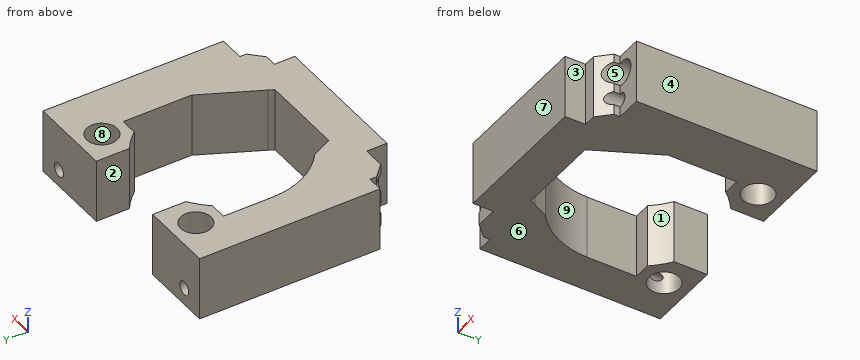
Autodesk Inventor part; units mm, degrees
ref_plane "YZ Plane" through (0, 0, 0) normal (1, 0, 0) x (0, 1, 0)
ref_plane "XZ Plane" through (0, 0, 0) normal (0, 1, 0) x (-1, 0, 0)
ref_plane "XY Plane" through (0, 0, 0) normal (0, 0, 1) x (1, 0, 0)
sketch "Sketch1" plane through (0, 0, 0) normal (0, 0, 1) x (1, 0, 0)
  line L0 (0, 0) -> (50, 0)
  line L1 (50, 0) -> (50, 36.921)
  line L2 (50, 36.921) -> (0, 36.921)
  line L3 (0, 36.921) -> (0, 0)
  dimension "d0" = 36.921
  dimension "d1" = 50
extrude "Extrusion1" add sketch "Sketch1" along normal blind 13
sketch "Sketch4" plane through (0, 0, 0) normal (0, 0, -1) x (-1, 0, 0)
  line L0 (-10, -8) -> (-40, -8)
  line L1 (-45.066, 0) -> (-2.934, 0)
  line L2 (-10.3, -8) -> (-10.3, -3.845)
  line L3 (-10.3, -3.845) -> (-5.7813, -3.845)
  line L4 (-5.7813, -3.845) -> (-3.234, -1.2977)
  line L5 (-3.234, -1.2977) -> (-3.234, 0)
  line L6 (-44.766, 0) -> (-44.766, -1.2977)
  line L7 (-44.766, -1.2977) -> (-42.2187, -3.845)
  line L8 (-42.2187, -3.845) -> (-39.7, -3.845)
  line L9 (-39.7, -3.845) -> (-39.7, -8)
  line L10 (0, 0) -> (-2.934, 0)
  line L11 (0, 0) -> (-50, 0)
  point P0 (-45.066, -1.422)
  dimension "d27" = 2.934
extrude "Extrusion4" add sketch "Sketch4" against normal blind 13
sketch "Sketch2" plane through (0, 0, 0) normal (0, -1, 0) x (1, 0, 0)
  circle A0 centre (44.9, 3.5) radius 1.4
  circle A1 centre (4.9, 3.5) radius 1.4
  line L0 (50, 0) -> (50, 13)
  circle A2 centre (45.7, 9) radius 2.5
  circle A3 centre (4.1, 9) radius 2.5
  line L1 (0, 0) -> (0, 13)
  line L2 (0, 13) -> (50, 13)
  dimension "d4" = 2.8
  dimension "d5" = 2.8
  dimension "d7" = 40
  dimension "d8" = 5
  dimension "d9" = 5
  dimension "d10" = 5.5
  dimension "d13" = 4.1
  dimension "d14" = 5.5
  dimension "d15" = 4
  dimension "d16" = 4.9
  dimension "d17" = 41.6
  dimension "d20" = 4
extrude "Extrusion2" cut sketch "Sketch2" along normal blind 10 and the other way blind 5
sketch "Sketch7" plane through (0, 0, 0) normal (0, 0, -1) x (-1, 0, 0)
  arc A0 (17, 30.1329) -> (13.5279, 26.921) centre (26, 16.921) ccw
  line L0 (10, 26.921) -> (13.5279, 26.921)
  line L1 (10, 12.8998) -> (10, 26.921)
  line L2 (15.8642, 1.1093) -> (10, 12.8998)
  line L3 (16.416, 0) -> (33.6258, 0)
  line L4 (16.416, 0) -> (15.8642, 1.1093)
  line L5 (34.1776, 1.1093) -> (33.6258, 0)
  line L6 (35.7354, 4.2414) -> (34.1776, 1.1093)
  arc A1 (35.7354, 4.2414) -> (41.9856, 16.8076) centre (26, 16.921) ccw
  line L7 (42, 26.921) -> (42, 16.8366)
  line L8 (38.4721, 26.921) -> (42, 26.921)
  arc A2 (38.4721, 26.921) -> (35, 30.1328) centre (26, 16.921) ccw
  line L9 (35, 36.921) -> (35, 30.1328)
  line L10 (17, 30.1329) -> (17, 36.921)
  circle A3 centre (11, 31.921) radius 3.1
  circle A4 centre (41, 31.921) radius 3.1
  line L11 (42, 16.8366) -> (41.9856, 16.8076)
  line L12 (17, 36.921) -> (35, 36.921)
  line L13 (17, 35.9386) -> (35, 35.9386)
  line L14 (35, 35.9386) -> (35, 37.4386)
  line L15 (35, 37.4386) -> (17, 37.4386)
  line L16 (17, 37.4386) -> (17, 35.9386)
  line L17 (0, 36.921) -> (0, 0)
  line L18 (0, 36.921) -> (-15, 36.921)
  line L19 (0, 36.921) -> (15, 36.921) construction
  line L20 (-33, 35.9386) -> (-15, 35.9386)
  line L21 (-33, 36.921) -> (-15, 36.921)
  line L22 (-15, 37.4386) -> (-33, 37.4386)
  line L23 (-33, 37.4386) -> (-33, 35.9386)
  line L24 (-33, 30.1329) -> (-33, 36.921)
  arc A5 (-33, 30.1329) -> (-36.4721, 26.921) centre (-24, 16.921) ccw
  circle A6 centre (-39, 31.921) radius 3.1
  line L25 (-40, 26.921) -> (-36.4721, 26.921)
  line L26 (-40, 12.8998) -> (-40, 26.921)
  line L27 (-34.1358, 1.1093) -> (-40, 12.8998)
  line L28 (-33.584, 0) -> (-16.3742, 0)
  line L29 (-33.584, 0) -> (-34.1358, 1.1093)
  line L30 (-8, 16.8366) -> (-8.0144, 16.8076)
  arc A7 (-14.2646, 4.2414) -> (-8.0144, 16.8076) centre (-24, 16.921) ccw
  line L31 (-14.2646, 4.2414) -> (-15.8224, 1.1093)
  line L32 (-15.8224, 1.1093) -> (-16.3742, 0)
  line L33 (-8, 26.921) -> (-8, 16.8366)
  line L34 (-15, 35.9386) -> (-15, 37.4386)
  arc A8 (-11.5279, 26.921) -> (-15, 30.1328) centre (-24, 16.921) ccw
  line L35 (-11.5279, 26.921) -> (-8, 26.921)
  circle A9 centre (-9, 31.921) radius 3.1
  line L36 (-15, 36.921) -> (-15, 30.1328)
  point P0 (-35, 36.921)
  dimension "d33" = 1.5
  dimension "d34" = 15
  dimension "d35" = 180
  dimension "d39" = 1.5
extrude "Extrusion7" cut sketch "Sketch7" against normal blind 13 contours L23 L21 L34 L20 | L20 L36 A8 L35 L33 L30 A7 L31 L32 L28 L29 L27 L26 L25 A5 L24 | L23 L22 L34 L21 | A6 | A9
sketch "Sketch8" plane through (0, 36.921, 13) normal (0, 1, 0) x (1, 0, 0)
  circle A0 centre (4.9, 9.5) radius 1.4
  circle A1 centre (44.9, 9.5) radius 1.4
  point P0 (0, 13)
extrude "Extrusion8" cut sketch "Sketch8" against normal blind 10
properties part number "30_CUBE_openSIM_Rodholder"
Design review of the part built by this model. Coordinates are the model's own, in mm. Face numbers are marked on the shaded views. A direction names the side the tool comes from. Coordinates: 2 decimals unless noted, no trailing zeros. Write each loop counter-clockwise with the first axis right and the second up, starting at its lowest first coordinate (ties: lowest second). Pieces come first, ordered by that corner, then holes. Notation, with made-up numbers: (-9, -35) - (19, -35) arc R32 cw to (19, -8) - close; hole circle Ø10 at (81, 0.5). An arc over 180 degrees is marked (long way). One line per item, written item: value.
1) Add section B-B (x = 13.5). State the section outline as (y, z) points, plus the area to 3 significant figures.
Answer sheet:
outline: (-8, 0) - (4.87, 0) - (4.87, 13) - (-8, 13) - close; (28.98, 0) - (36.92, 0) - (36.92, 13) - (28.98, 13) - close
area: 271 mm2
2) Add section C-C (x = 45.7). State the section outline as (y, z) points.
Answer sheet:
outline: (0, 0) - (36.92, 0) - (36.92, 2.35) - (26.92, 2.35) - (26.92, 4.65) - (36.92, 4.65) - (36.92, 13) - (0, 13) - (0, 11.5) - (5, 11.5) - (5, 6.5) - (0, 6.5) - (0, 4.65) - (5, 4.65) - (5, 2.35) - (0, 2.35) - close
3) To check wall thickness, follow probe 1 along X at (y, z) = (17.5, 8.75); probe 2 along Y at (x, z) = (11, 7); probe 3 along Y at (x, z) = (39, 4.5). State the ranges of each line that lie inside material, in increasing order.
Answer sheet:
probe 1: x = 0 to 8, 40 to 50
probe 2: y = -8 to 7.62, 26.92 to 29.55, 34.29 to 36.92
probe 3: y = -8 to 10.89, 26.92 to 28.82, 35.02 to 36.92
4) Add section D-D (x = 4.9). State the section outline as (y, z) points, plus the area to 3 significant figures.
Answer sheet:
outline: (-2.96, 0) - (36.92, 0) - (36.92, 2.1) - (26.92, 2.1) - (26.92, 4.9) - (36.92, 4.9) - (36.92, 13) - (-2.96, 13) - (-2.96, 11.37) - (5, 11.37) - (5, 6.63) - (-2.96, 6.63) - (-2.96, 4.9) - (5, 4.9) - (5, 2.1) - (-2.96, 2.1) - close
area: 430 mm2
5) Insertion check: pin 1 (2.5 mm diameter, centred on x = 3.5, z = 10, fed in from -Y); pin 2 (1 mm diameter, centred on x = 29.5, z = 2.5, fed in from +Y); pin 3 (2 mm diameter, centred on x = 4.9, z = 3.5, fed in from +Y). Each pin has a flat end and moves straight along its axis. Give the tip position at first contact, or say it passes through.
Answer sheet:
pin 1: stops at y = 5
pin 2: stops at y = 0
pin 3: stops at y = 26.92
6) Add section A-A (y = 21). State the section outline as (x, z) points, plus the area to 3 significant figures.
Answer sheet:
outline: (0, 0) - (8, 0) - (8, 13) - (0, 13) - close; (40, 0) - (50, 0) - (50, 13) - (40, 13) - close
area: 234 mm2
7) Mouldability with a two-part tool opening along Y and no side actions: class the marked faces 6, 7, 8 and 9 as +Y half, -Y half, draft (parallel to the pull), parting line (faces both ways), or undercut.
Answer sheet:
face 6: draft
face 7: -Y half
face 8: undercut
face 9: undercut
8) For the marked faces 1, 2, 3, 4 and 5, list the 3-axis set-ups (+Z, -Z, +X, -X, +Y, -Y) from which the entire face can be reached by the end or side of a thin tool; tool diameter is ignored.
Answer sheet:
face 1: +Z, -Z
face 2: +Z, -Z, +Y
face 3: +Z, -Z, +X, -Y
face 4: +Z, -Z, +X, +Y, -Y
face 5: -Y
